Job drawing, mm, ordinate dimensions from the low corner. One solid piece. A direction names the side the tool comes from. Give positions to 0.01 mm unless a question says otherwise; leave off trailing zeros. Order: outer loops, then holes, each group sorted by start corner. A loop starts at its lowest first (then second) coordinate and runs counter-clockwise, first axis right, second up. Notation, with made-up numbers: (87.5, -1) -> (127.5, -1) arc R18 ccw to (127.5, 30) -> close; hole circle Ø1 at (48.25, -7). An arc over 180 degrees is marked (long way). Write item = value, one per line. Start each with the question number.
(1) Which spindle directions (+Z, -Z, +X, -X, +Y, -Y) get a long thin tool onto all of the face, cutting with end or side? Do the marked faces 4 and 5. Say none if no direction does.
(2) Two-plate mould, pull along Y, no slides. Class the marked faces 1, 2 and 3: pulls with the +Y half, pulls with the -Y half, needs draft (parallel to the pull), parting line crosses it, or undercut.
(3) Saw through at D-D, the plane x = 8. List the corners of the cut face in (y, z).
(4) Saw through at A-A, the plane y = 12.5. List the corners of the cut face in (x, z) (3 decimals).
(5) Saw through at C-C, the plane z = 2.75. List the corners of the cut face in (x, y) (3 decimals).
(6) Flat gauge pins, fed straight in: pin 1 (5 mm diameter, centred on y = 17.5, z = 3, fed in from -X); pin 2 (2 mm diameter, centred on x = 18.5, z = 7, fed in from +Y); pin 3 (4 mm diameter, centred on x = 7.5, y = 8.5, fed in from +Z); pin 4 (2 mm diameter, centred on x = 12, y = 14, fed in from +Z). Where does each tip first touch, or does it go through?
(7) Probe line 1 along Y through (x, z) = (12.5, 5.75); line 2 along Y through (x, z) = (13.75, 3.5); line 3 along X through (y, z) = (13.5, 2.75). List the from-to ranges inside material, lowest first. Write a range as from..to.
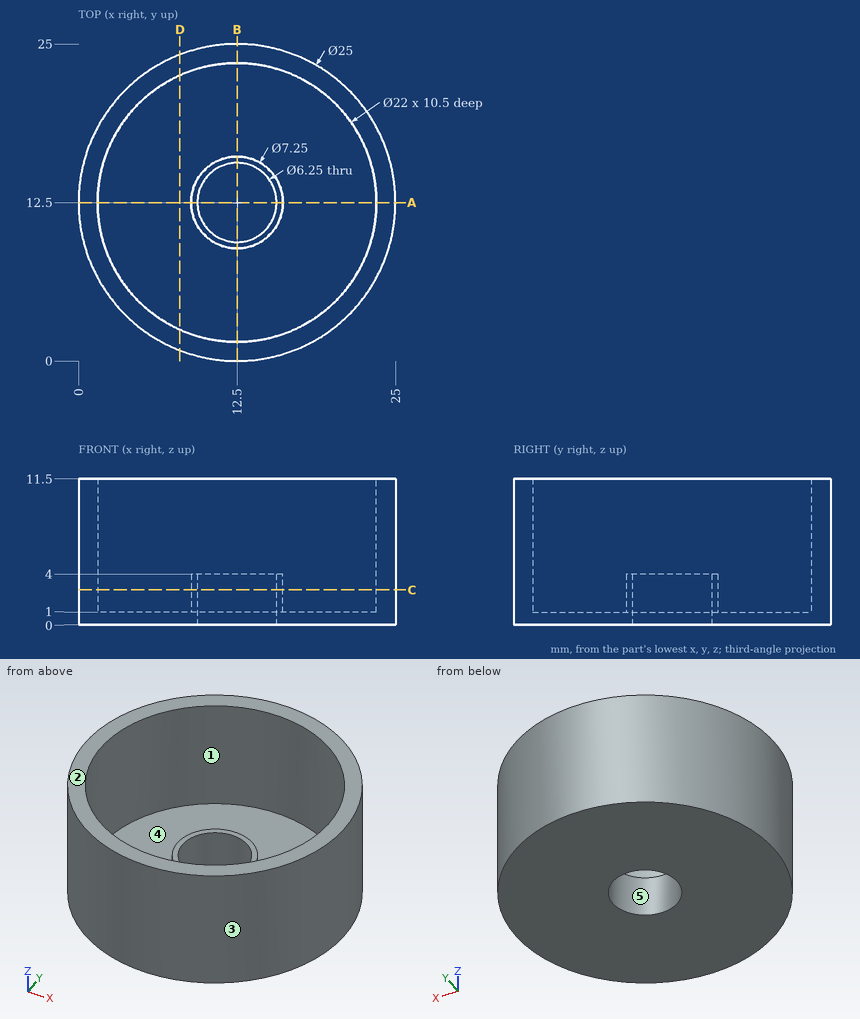
Results list:
q1.face_4 = +Z
q1.face_5 = +Z, -Z
q2.face_1 = undercut
q2.face_2 = needs draft
q2.face_3 = parting line crosses it
q3.outline = (0.84, 0) -> (24.16, 0) -> (24.16, 11.5) -> (22.54, 11.5) -> (22.54, 1) -> (2.46, 1) -> (2.46, 11.5) -> (0.84, 11.5) -> close
q4.outline = (0, 0) -> (9.375, 0) -> (9.375, 4) -> (8.875, 4) -> (8.875, 1) -> (1.5, 1) -> (1.5, 11.5) -> (0, 11.5) -> close; (15.625, 0) -> (25, 0) -> (25, 11.5) -> (23.5, 11.5) -> (23.5, 1) -> (16.125, 1) -> (16.125, 4) -> (15.625, 4) -> close
q5.outline = circle Ø25 at (12.5, 12.5); circle Ø7.25 at (12.5, 12.5); hole circle Ø22 at (12.5, 12.5); hole circle Ø6.25 at (12.5, 12.5)
q6.pin_1 = 0.25
q6.pin_2 = 23.96
q6.pin_3 = 1
q6.pin_4 = through
q7.line_1 = 0..1.5, 23.5..25
q7.line_2 = 0.06..1.57, 9.1..9.64, 15.36..15.9, 23.43..24.94
q7.line_3 = 0.04..1.55, 9.02..9.54, 15.46..15.98, 23.45..24.96
